```python
from build123d import *

# Parameters (mm, degrees)
F0_R     = 14.4
F0_R_2   = 10.75
F1_DEPTH = 61.8
F2_R     = 14.4
F2_R_2   = 10.75
F3_DEPTH = 27.5
F5_D     = 8
F5_DEPTH = 14.401


with BuildPart() as f1:
    # F0 (on Front) → F1 (new body)
    with BuildSketch(Plane.XZ):
        Circle(F0_R)
        Circle(F0_R_2, mode=Mode.SUBTRACT)
    extrude(amount=F1_DEPTH)

    # F2 (on Top) → F3 (join)
    with BuildSketch(Plane.XY):
        with Locations((0, -30.9)):
            Circle(F2_R)
        with Locations((0, -30.9)):
            Circle(F2_R_2, mode=Mode.SUBTRACT)
    extrude(amount=F3_DEPTH)

    # F5 (through all, one way)
    with BuildSketch(Plane.XY):
        with Locations((0, -30.9)):
            Circle(F5_D / 2)
    extrude(amount=-F5_DEPTH, mode=Mode.SUBTRACT)


solid = f1.part
```
Source: CAD feature listing. Evaluate the final solid. Frame: model axes, mm. A direction names the side the tool comes from. Give positions to 0.01 mm unless a question says otherwise; leave off trailing zeros. Loops run counter-clockwise (first coordinate to the right, second up) from the corner with the lowest first, then second, coordinate; pieces in that order, holes last. Notation, with made-up numbers: (6, 86.5) -> (40, 86.5) arc R27 ccw to (40, 122.5) -> close; hole circle Ø7 at (31, 20.5). An arc over 180 degrees is marked (long way). Use a Markdown table: item, result. Add a question column.
(1) Section query B-B (y = -18.5). Output: boundary loops of the cut face in (x, z), then the cut area to 3 significant figures.
(2) Access query for faces 1 (the face through (3.695, -32.432, -12.158)), 2 (the face through (-10.613, -21.168, 16.613)), 3 (the face through (0.236, -30.75, 10.747)), 4 (the face through (-0.1, -19.9, 0)). Directions: +Z, -Z, +X, -X, +Y, -Y. A direction counts if a zero-diameter tool reaches every point of the face in a straight line with its end or side. Return the directions, or none.
(3) First-contact query: pin 1 Ø2 at (x, y) = (11, -16.5) entering from +Z; pin 2 Ø1 at (y, z) = (-30.5, -7.5) entering from +X; pin 3 Ø5 at (x, z) = (1.5, 7) entering from +Y. Flat tips, straight axial feed; report the tip coordinate or a pass-through.
(4) Pull-direction query (Z, two-part tool) for faces 5 (the face through (-1, -42, 0)), 6 (the face through (6.6, -30.5, -12.8)), 7 (the face through (9.93, -35.02, 20.41)); classes: +Z half, -Z half, draft (parallel to the pull), parting line (faces both ways), or undercut.
(5) Section query A-A (x = 0). Output: boundary loops of the cut face in (y, z).
(6) Section query C-C (z = -2). Output: boundary loops of the cut face in (x, y), then the cut area to 3 significant figures.
(7) Ray query, line 1 (Z direction, x = 0, y = -8); line 2 (Y direction, x = 0, z = -11.95). Return the intervals inside material, ascending.
(8) Section query D-D (z = 5). Output: boundary loops of the cut face in (x, y), then the cut area to 3 significant figures.
Checked values:
| question | item | result |
|---|---|---|
| 1 | outline | (-7.32, 12.4) arc R14.4 ccw (long way) to (7.32, 12.4) -> (7.32, 27.5) -> (-7.32, 27.5) -> close; hole (-7.32, 0) -> (-7.32, 7.87) arc R10.75 ccw (long way) to (7.32, 7.87) -> (7.32, 0) -> close |
| 1 | area | 634 mm^2 |
| 2 | face 1 | -Z |
| 2 | face 2 | +Z |
| 2 | face 3 | none |
| 2 | face 4 | +Y, -Y |
| 3 | pin 1 | z = 10.36 |
| 3 | pin 2 | x = 12.58 |
| 3 | pin 3 | y = -16.5 |
| 4 | face 5 | undercut |
| 4 | face 6 | parting line |
| 4 | face 7 | draft |
| 5 | outline | (-61.8, -14.4) -> (-34.9, -14.4) -> (-34.9, -10.75) -> (-61.8, -10.75) -> close; (-61.8, 10.75) -> (-45.3, 10.75) -> (-45.3, 0) -> (-41.65, 0) -> (-41.65, 10.75) -> (-20.15, 10.75) -> (-20.15, 0) -> (-16.5, 0) -> (-16.5, 10.75) -> (0, 10.75) -> (0, 14.4) -> (-16.5, 14.4) -> (-16.5, 27.5) -> (-20.15, 27.5) -> (-20.15, 14.4) -> (-41.65, 14.4) -> (-41.65, 27.5) -> (-45.3, 27.5) -> (-45.3, 14.4) -> (-61.8, 14.4) -> close; (-26.9, -14.4) -> (0, -14.4) -> (0, -10.75) -> (-26.9, -10.75) -> close |
| 6 | outline | (-14.26, -61.8) -> (-10.56, -61.8) -> (-10.56, 0) -> (-14.26, 0) -> close; (10.56, -61.8) -> (14.26, -61.8) -> (14.26, 0) -> (10.56, 0) -> close |
| 6 | area | 457 mm^2 |
| 7 | line 1 | -14.4 to -10.75, 10.75 to 14.4 |
| 7 | line 2 | -61.8 to -34.9, -26.9 to 0 |
| 8 | outline | (-13.5, -61.8) -> (-9.52, -61.8) -> (-9.52, -41.71) arc R14.4 ccw to (9.52, -41.71) -> (9.52, -61.8) -> (13.5, -61.8) -> (13.5, -35.9) arc R14.4 ccw to (13.5, -25.9) -> (13.5, 0) -> (9.52, 0) -> (9.52, -20.09) arc R14.4 ccw to (-9.52, -20.09) -> (-9.52, 0) -> (-13.5, 0) -> (-13.5, -25.9) arc R14.4 ccw to (-13.5, -35.9) -> close; hole (-9.52, -35.9) arc R10.75 ccw to (9.52, -35.9) -> (9.52, -25.9) arc R10.75 ccw to (-9.52, -25.9) -> close |
| 8 | area | 664 mm^2 |
